```python
from build123d import *
from build123d.topology import SkipClean

# Parameters (mm, degrees)
BOSS_EXTRUDE1_DEPTH = 38
BOSS_EXTRUDE2_REACH = 81.624
CUT_EXTRUDE1_START  = -38
SKETCH3_R           = 27
CUT_EXTRUDE1_DEPTH  = 38
SKETCH4_R           = 4.5
CUT_EXTRUDE2_DEPTH  = 64
CUT_EXTRUDE3_DEPTH  = 64


with BuildPart() as part:
    # Sketch1 → Boss-Extrude1 (new body)
    with BuildSketch(Plane.XY):
        with BuildLine():
            ThreePointArc((36, 0), (0, 36), (-36, 0))
            Line((-36, 0), (-27, 0))
            ThreePointArc((-27, 0), (0, 27), (27, 0))
            Line((27, 0), (36, 0))
        make_face()
    extrude(amount=BOSS_EXTRUDE1_DEPTH)

    # Boss-Extrude2: up to this face of the body (flat: up to its plane)
    boss_extrude2_end = Plane(part.part.faces().sort_by_distance((31.5, 0, 19))[0])
    # Sketch2 → Boss-Extrude2 (add, up to the picked face)
    with BuildSketch(Plane(origin=(0, 60, 0), x_dir=(-1, 0, 0), z_dir=(0, -1, 0)), mode=Mode.PRIVATE) as boss_extrude2_sk1:
        with BuildLine():
            Line((-39.272787465, -10), (39.272787465, -10))
            ThreePointArc((39.272787465, -10), (48.272787465, -19), (39.272787465, -28))
            Line((39.272787465, -28), (-39.272787465, -28))
            ThreePointArc((-39.272787465, -28), (-48.272787465, -19), (-39.272787465, -10))
        make_face()
    boss_extrude2_tool1 = split(extrude(boss_extrude2_sk1.sketch, amount=BOSS_EXTRUDE2_REACH, mode=Mode.PRIVATE), bisect_by=boss_extrude2_end, keep=Keep.BOTH, mode=Mode.PRIVATE)
    add(boss_extrude2_tool1.solids().sort_by(Axis((0, 60, 19), (0, -1, 0)))[0])

    # Sketch3 → Cut-Extrude1 (cut)
    with SkipClean():  # the faces are left unmerged after this step: merging them gives an invalid solid
        with BuildSketch(Plane.XY.offset(28).offset(CUT_EXTRUDE1_START)):
            Circle(SKETCH3_R)
        extrude(amount=CUT_EXTRUDE1_DEPTH, mode=Mode.SUBTRACT)
    add(part.part.scale(1), mode=Mode.REPLACE)  # the faces are merged on a copy

    # Sketch4 → Cut-Extrude2 (cut)
    with BuildSketch(Plane(origin=(0, 60, 0), x_dir=(1, 0, 0), z_dir=(0, 1, 0))):
        with Locations(Location((-39.272787465, -19, 0), (0, 0, 270))):
            Circle(SKETCH4_R)
    cut_extrude2 = extrude(amount=-CUT_EXTRUDE2_DEPTH, mode=Mode.SUBTRACT)

    # Mirror1: Cut-Extrude2 across plane
    add(cut_extrude2.mirror(Plane(origin=(0, 0, 0), x_dir=(0, 0, 1), z_dir=(1, 0, 0))), mode=Mode.SUBTRACT)

    # Sketch6 → Cut-Extrude3 (cut)
    with BuildSketch(Plane.XY.offset(28)):
        Polygon((-48.272787465, 40), (-39.272787465, 47.2), (-39.272787465, 60), (-48.272787465, 60), align=None)
        Polygon((-39.272787465, 47.2), (-23.272787465, 60), (-39.272787465, 60), align=None)
    cut_extrude3 = extrude(amount=-CUT_EXTRUDE3_DEPTH, mode=Mode.SUBTRACT)

    # Mirror2: Cut-Extrude3 across plane
    add(cut_extrude3.mirror(Plane(origin=(0, 0, 0), x_dir=(0, 0, 1), z_dir=(1, 0, 0))), mode=Mode.SUBTRACT)


solid = part.part
```
Geometry: final body of the model. Coordinates: model frame, mm. A direction names the side the tool comes from. Round coordinates to 2 decimals unless told otherwise and drop trailing zeros. Loops run counter-clockwise (first coordinate to the right, second up) from the corner with the lowest first, then second, coordinate; pieces in that order, holes last. Notation, with made-up numbers: (3.5, 57) -> (8.5, 57) arc R25 ccw to (8.5, 88) -> close; hole circle Ø11 at (82, 52.25). An arc over 180 degrees is marked (long way). Use one line per item in the form item = value.
Item 1: Cut plane A-A on y = 22. Output: boundary loops of the cut face in (x, z).
Evaluation:
outline = (-39.27, 10) -> (-28.5, 10) -> (-28.5, 0) -> (-15.65, 0) -> (-15.65, 38) -> (-28.5, 38) -> (-28.5, 28) -> (-39.27, 28) arc R9 ccw to start; (15.65, 0) -> (28.5, 0) -> (28.5, 10) -> (39.27, 10) arc R9 ccw to (39.27, 28) -> (28.5, 28) -> (28.5, 38) -> (15.65, 38) -> close; hole circle Ø9 at (-39.27, 19); hole circle Ø9 at (39.27, 19)
Item 2: Draft query along X for faces 1 (the cylindrical face through (34.81, 25.76, 18.41)), 2 (the cylindrical face through (-48.27, 23.93, 18.8)), 3 (the cylindrical face through (0.79, 35.99, 4.93)). Return one class per face: released by +X, released by -X, zero draft, split by the parting line, or undercut.
Evaluation:
face_1 = undercut
face_2 = released by -X
face_3 = split by the parting line
Item 3: Material intervals for probe 1 along Z at (x, y) = (-26, 47); probe 2 along X at (y, z) = (23.5, 19); probe 3 along X at (y, z) = (2, 22), sorted ascending.
Evaluation:
probe_1 = 10 to 28
probe_2 = -48.27 to -43.77, -34.77 to -13.29, 13.29 to 34.77, 43.77 to 48.27
probe_3 = -47.76 to -42.63, -35.92 to -26.93, 26.93 to 35.92, 42.63 to 47.76
Item 4: Access query for faces 4 (the cylindrical face through (0.79, 35.99, 32.93)), 5 (the flat face through (33.17, 52.08, 19.13)). Directions: +Z, -Z, +X, -X, +Y, -Y. A direction counts if a zero-diameter tool reaches every point of the face in a straight line with its end or side. Return the directions, or none.
Evaluation:
face_4 = +Z, +Y
face_5 = +Z, -Z, +X, +Y
Item 5: Cut plane D-D on y = 30.5. Output: boundary loops of the cut face in (x, z).
Evaluation:
outline = (-39.27, 10) -> (-19.12, 10) -> (-19.12, 0) -> (19.12, 0) -> (19.12, 10) -> (39.27, 10) arc R9 ccw to (39.27, 28) -> (19.12, 28) -> (19.12, 38) -> (-19.12, 38) -> (-19.12, 28) -> (-39.27, 28) arc R9 ccw to start; hole circle Ø9 at (-39.27, 19); hole circle Ø9 at (39.27, 19)
Item 6: Cut plane B-B on z = 19. Output: boundary loops of the cut face in (x, y), then the cut area to 3 significant figures.
Evaluation:
outline = (-48.27, 0) -> (-43.77, 0) -> (-43.77, 43.6) -> (-48.27, 40) -> close; (-34.77, 0) -> (-27, 0) arc R27 cw to (27, 0) -> (34.77, 0) -> (34.77, 50.8) -> (23.27, 60) -> (-23.27, 60) -> (-34.77, 50.8) -> close; (43.77, 0) -> (48.27, 0) -> (48.27, 40) -> (43.77, 43.6) -> close
area = 3,300 mm2
Item 7: Cut plane C-C on x = 0. Output: boundary loops of the cut face in (y, z), then the cut area to 3 significant figures.
Evaluation:
outline = (27, 0) -> (36, 0) -> (36, 10) -> (60, 10) -> (60, 28) -> (36, 28) -> (36, 38) -> (27, 38) -> close
area = 774 mm2
Item 8: Contact query for flat-ended pins moving along their axis: pin 1 Ø4 at (x, y) = (8.5, 46.5) entering from -Z; pin 2 Ø10 at (y, z) = (29.5, 10.5) entering from -X; pin 3 Ø4 at (y, z) = (35.5, 12) entering from -X. Output: stop coordinate, or through.
Evaluation:
pin_1 = 10
pin_2 = -47.56
pin_3 = -46.76
